The drawing under review shows one solid part. Ordinate dimensions are in mm from its lowest x, y, z. A direction names the side the tool comes from. Coordinates: 2 decimals unless noted, no trailing zeros. Order: outer loops, then holes, each group sorted by start corner. A loop starts at its lowest first (then second) coordinate and runs counter-clockwise, first axis right, second up.
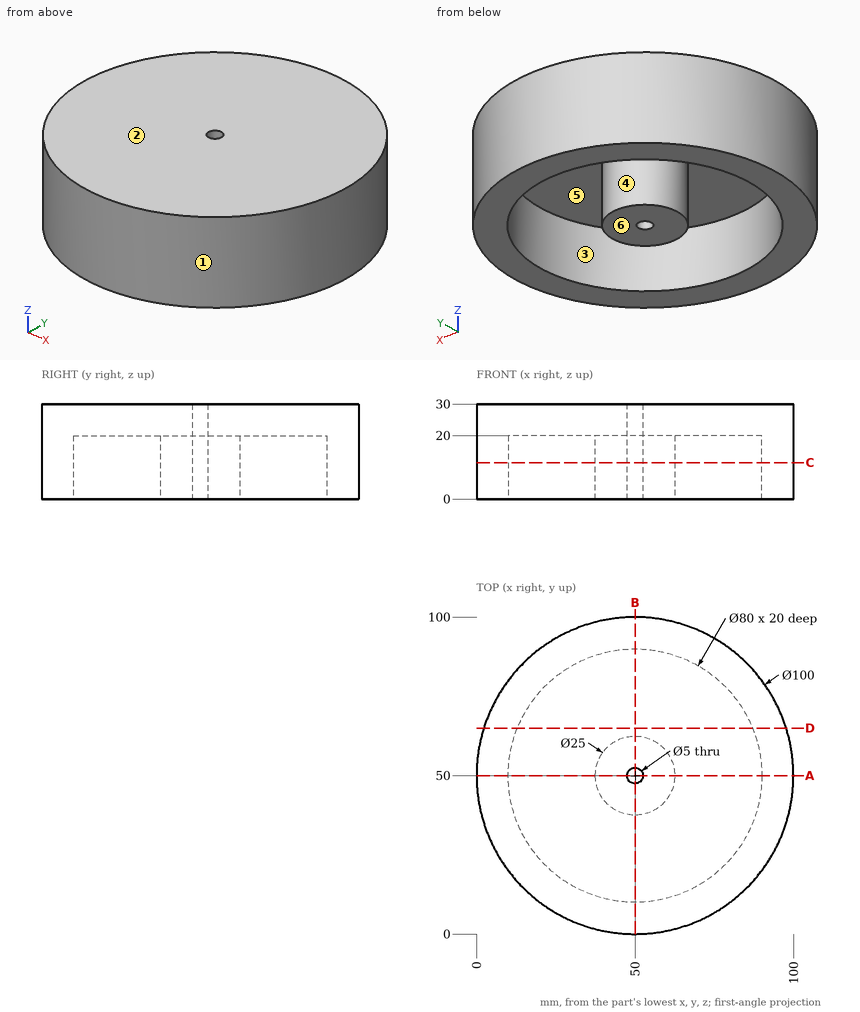
(1) We need section A-A, the plane y = 50. Write out the cut boundary in (x, z).
A:
outline: (0, 0) - (10, 0) - (10, 20) - (37.5, 20) - (37.5, 0) - (47.5, 0) - (47.5, 30) - (0, 30) - close; (52.5, 0) - (62.5, 0) - (62.5, 20) - (90, 20) - (90, 0) - (100, 0) - (100, 30) - (52.5, 30) - close
(2) For pin 1 Ø1.5 at (x, z) = (17, 17.5) entering from -Y; pin 2 Ø5 at (x, z) = (60, 17) entering from +Y; pin 3 Ø1 at (x, y) = (62, 18) entering from -Z, all flat-tipped, find the tip position at first contact; note any pin that passes through.
A:
pin 1: stops at y = 11.79
pin 2: stops at y = 99.43
pin 3: stops at z = 20
(3) Wall thickness on probe 1 along Y at (x, z) = (50, 15.25); probe 2 along X at (y, z) = (54.5, 19.25); probe 3 along X at (y, z) = (34.5, 10): over which ranges is each line inside the solid? List them lowest first.
A:
probe 1: y = 0 to 10, 37.5 to 47.5, 52.5 to 62.5, 90 to 100
probe 2: x = 0.2 to 10.25, 38.34 to 61.66, 89.75 to 99.8
probe 3: x = 2.46 to 13.13, 86.87 to 97.54
(4) We need section C-C, the plane z = 11.5. Write out the cut boundary in (x, y), and give its area (3 significant figures).
A:
outline: circle Ø100 at (50, 50); circle Ø25 at (50, 50); hole circle Ø80 at (50, 50); hole circle Ø5 at (50, 50)
area: 3,300 mm2
(5) Machinability: for the marked faces 5 and 6, which of the approach directions +Z, -Z, +X, -X, +Y, -Y give a long, thin tool a straight path to every point of the face, cutting with its end or side? Answer none if there is none.
A:
face 5: -Z
face 6: -Z, +X, -X, +Y, -Y
(6) Draft analysis for pull direction Y (two halves, no side actions). For the marked faces 1, 2, 3 and 4, state which applies: released by +Y, released by -Y, zero draft, split by the parting line, or undercut.
A:
face 1: split by the parting line
face 2: zero draft
face 3: undercut
face 4: undercut
(7) We need section D-D, the plane y = 65. Write out the cut boundary in (x, z).
A:
outline: (2.3, 0) - (12.92, 0) - (12.92, 20) - (87.08, 20) - (87.08, 0) - (97.7, 0) - (97.7, 30) - (2.3, 30) - close
